Geometry check sheet. Reference: the model listing, model coordinates, mm. A direction names the side the tool comes from. Coordinates: 2 decimals unless noted, no trailing zeros. Loops run counter-clockwise (first coordinate to the right, second up) from the corner with the lowest first, then second, coordinate; pieces in that order, holes last.
from build123d import *

# Parameters (mm, degrees)
F0_W     = 45.72
F0_H     = 30.48
F1_DEPTH = 0.6985
F2_W     = 15.24
F2_H     = 15.24
F3_DEPTH = 1.398
F4_W     = 15.24
F4_H     = 1.397
F5_DEPTH = 24.003
F6_R     = 2.3876
F7_DEPTH = 1.398


with BuildPart() as f1:
    # F0 (on Front) → F1 (new body, symmetric)
    with BuildSketch(Plane.XZ):
        Rectangle(F0_W, F0_H)
    extrude(amount=F1_DEPTH, both=True)

    # F2 (on face) → F3 (cut, through all)
    with BuildSketch(Plane.XZ.offset(0.6985)):
        with Locations((-15.24, -7.62)):
            Rectangle(F2_W, F2_H)
        with Locations((15.24, -7.62)):
            Rectangle(F2_W, F2_H)
    extrude(amount=-F3_DEPTH, mode=Mode.SUBTRACT)

    # F4 (on face) → F5 (join)
    with BuildSketch(Plane.XZ.offset(0.6985)):
        with Locations((0, -14.5415)):
            Rectangle(F4_W, F4_H)
    extrude(amount=F5_DEPTH)

    # F6 (on face) → F7 (cut, through all)
    with BuildSketch(Plane.XY.offset(-13.843)):
        with Locations((0, -18.3515)):
            Circle(F6_R)
    extrude(amount=-F7_DEPTH, mode=Mode.SUBTRACT)


solid = f1.part
(1) Sectioned sample at C-C on x = -6.5. Record the cut outline in (y, z), and give its area (3 significant figures).
Findings:
outline: (-24.7, -15.24) - (0.7, -15.24) - (0.7, 15.24) - (-0.7, 15.24) - (-0.7, -13.84) - (-24.7, -13.84) - close
area: 76.1 mm2
(2) Sectioned sample at D-D on z = -0.5. Record the cut outline in (x, y).
Findings:
outline: (-7.62, -0.7) - (7.62, -0.7) - (7.62, 0.7) - (-7.62, 0.7) - close
(3) Access from +Z, -Z, +X, -X, +Y, -Y to the whole of each face (thin tool, end or side, straight path). Record for faces 5 (the flat face through (-15, 0, 0)), 6 (the flat face through (0, -13, -13.843)), 7 (the flat face through (7.62, -8, -14)), 8 (the flat face through (0, 0, 15.24)).
Findings:
face 5: -Z, -X, +Y, -Y
face 6: +Z, +X, -X, -Y
face 7: -Z, +X, +Y, -Y
face 8: +Z, +X, -X, +Y, -Y
(4) Gauge pin test, flat ends, axial feed: pin 1 Ø1.5 at (x, y) = (-16.5, -0.5) entering from -Z; pin 2 Ø2 at (x, y) = (-17, -2.5) entering from +Z; pin 3 Ø5.5 at (x, y) = (0, -18.35) entering from +Z; pin 4 Ø8 at (y, z) = (-18.5, -10.5) entering from -X. Record the tip position at first contact, or that the pin passes through.
Findings:
pin 1: stops at z = 0
pin 2: passes through
pin 3: stops at z = -13.84
pin 4: stops at x = -7.62
(5) Scan lines: L1, parallel to Y at x = 0, z = -14; L2, parallel to Z at x = -6, y = -14.25; L3, parallel to Z at x = -12.5, y = -0.5. Record each from-to range of solid material in increasing order.
Findings:
L1: y = -24.7 to -20.74, -15.96 to 0.7
L2: z = -15.24 to -13.84
L3: z = 0 to 15.24
(6) Draft check along X on faces 1 (the flat face through (22.86, 0, 8)), 2 (the flat face through (-7.62, -8, -14)), 3 (the flat face through (0, -12, -15.24)), 4 (the cylindrical face through (-0.52, -20.68, -14.53)). Enter one of: +X half, -X half, draft (parallel to the pull), parting line (faces both ways), or undercut.
Findings:
face 1: +X half
face 2: -X half
face 3: draft
face 4: undercut
(7) Sectioned sample at B-B on y = -17.75. Record the cut outline in (x, z), and give its area (3 significant figures).
Findings:
outline: (-7.62, -15.24) - (-2.31, -15.24) - (-2.31, -13.84) - (-7.62, -13.84) - close; (2.31, -15.24) - (7.62, -15.24) - (7.62, -13.84) - (2.31, -13.84) - close
area: 14.8 mm2
(8) Sectioned sample at A-A on x = 0. Record the cut outline in (y, z), and give its area (3 significant figures).
Findings:
outline: (-24.7, -15.24) - (-20.74, -15.24) - (-20.74, -13.84) - (-24.7, -13.84) - close; (-15.96, -15.24) - (0.7, -15.24) - (0.7, 15.24) - (-0.7, 15.24) - (-0.7, -13.84) - (-15.96, -13.84) - close
area: 69.4 mm2
